For this review, use the dimensioned drawing (mm, ordinates from the lowest corner) and the shaded views. A direction names the side the tool comes from. Give positions to 0.01 mm unless a question says otherwise; leave off trailing zeros. Loops run counter-clockwise (first coordinate to the right, second up) from the corner with the lowest first, then second, coordinate; pieces in that order, holes last. Notation, with made-up numbers: (19, -1.75) -> (66, -1.75) arc R21 cw to (66, 27.25) -> close; hole circle Ø6 at (24.25, 88). An arc over 180 degrees is marked (long way). Write each question's results on one line, items separated by ' | '. Start each with the question number.
Q1. Machinability: for the marked faces 1, 2 and 3, which of the approach directions +Z, -Z, +X, -X, +Y, -Y give a long, thin tool a straight path to every point of the face, cutting with its end or side? Answer none if there is none.
Q2. We need section A-A (x = 11). Write out the cut boundary in (y, z).
Q3. We need section D-D (y = 9.5). Write out the cut boundary in (x, z).
Q4. We need section B-B (z = 11). Write out the cut boundary in (x, y).
Q5. Wall thickness on L1, parallel to X at y = 7, z = 11; L2, parallel to X at y = 3.5, z = 11; L3, parallel to Y at x = 20.5, z = 9.75: over which ranges is each line inside the solid? List them lowest first. Write a range as [from, to].
Q6. Insertion check: pin 1 Ø2 at (y, z) = (9.5, 6) entering from +X; pin 2 Ø1 at (y, z) = (6, 13) entering from +X; pin 3 Ø2 at (y, z) = (4.5, 16.5) entering from +X. Each pin has a flat end and moves straight along its axis. Give the tip position at first contact, or say it passes through.
Q7. We need section C-C (y = 5.75). Write out the cut boundary in (x, z), plus the area to 3 significant figures.
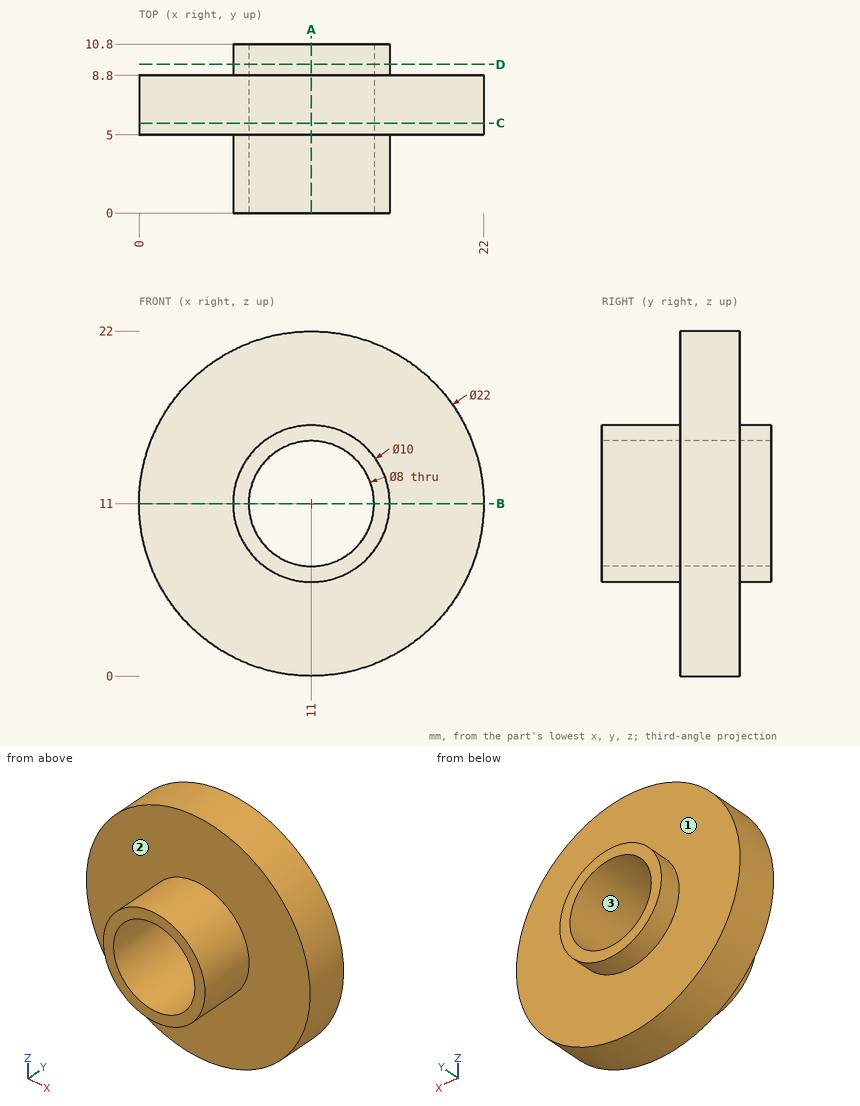
Output:
1) face 1: +Y | face 2: -Y | face 3: +Y, -Y
2) outline: (0, 6) -> (5, 6) -> (5, 0) -> (8.8, 0) -> (8.8, 6) -> (10.8, 6) -> (10.8, 7) -> (0, 7) -> close; (0, 15) -> (10.8, 15) -> (10.8, 16) -> (8.8, 16) -> (8.8, 22) -> (5, 22) -> (5, 16) -> (0, 16) -> close
3) outline: circle Ø10 at (11, 11); hole circle Ø8 at (11, 11)
4) outline: (0, 5) -> (6, 5) -> (6, 0) -> (7, 0) -> (7, 10.8) -> (6, 10.8) -> (6, 8.8) -> (0, 8.8) -> close; (15, 0) -> (16, 0) -> (16, 5) -> (22, 5) -> (22, 8.8) -> (16, 8.8) -> (16, 10.8) -> (15, 10.8) -> close
5) L1: [0, 7], [15, 22] | L2: [6, 7], [15, 16] | L3: [5, 8.8]
6) pin 1: x = 21.13 | pin 2: x = 21.9 | pin 3: x = 20.98
7) outline: circle Ø22 at (11, 11); hole circle Ø8 at (11, 11) | area: 330 mm2
